Geometry: final body of the model. Coordinates: model frame, mm. Face numbers are marked on the shaded views. A direction names the side the tool comes from. Give positions to 0.01 mm unless a question says otherwise; leave off trailing zeros. Write each loop counter-clockwise with the first axis right and the second up, starting at its lowest first coordinate (ties: lowest second). Pieces come first, ordered by that corner, then holes.
Q1. Mould query, pull axis Z, two halves, no side actions, for the marked faces 6, 7, 8 and 9. Classes: +Z half, -Z half, draft (parallel to the pull), parting line (faces both ways), or undercut.
Q2. Reachability of the marked faces 1, 2, 3, 4 and 5 from +Z, -Z, +X, -X, +Y, -Y: full face, straight path, thin tool, end or side. Return the list, or none.
Q3. Section A-A (x = 26.75). Return the cut outline in (y, z).
Q4. Line query: line 1 (Z direction, x = 23, y = 8.75); line 2 (Z direction, x = 24, y = 20.25); line 3 (Y direction, x = 3.25, z = 5.75). Output: solid intervals per line, ascending.
Q5. Section C-C (x = 17). Return the cut outline in (y, z) (3 decimals).
Q6. Section B-B (y = 2.5). State how many separate pieces and enclosed holes the cut face has, plus the area to 3 significant figures.
Q7. Pin query (flat end, axial travel): pin 1 Ø2 at (y, z) = (16, 3) entering from -X; pin 2 Ø1.5 at (y, z) = (5, 4) entering from +X; pin 3 Ø0.7 at (x, y) = (15.5, 9) entering from -Z. Return the tip coordinate at first contact, or that it passes through.
from build123d import *

# Parameters (mm, degrees)
SKETCH_W             = 28
SKETCH_H             = 22
PAD002_DEPTH         = 5
POCKET001_DEPTH      = 0.8
SKETCH002_W          = 0.6
SKETCH002_H          = 23
POCKET_DEPTH         = 4
LINEARPATTERN_COUNT  = 9
LINEARPATTERN_PITCH  = 2.375
POCKET002_DEPTH      = 3.5
SKETCH006_W          = 28
SKETCH006_H          = 22
POCKET005_DEPTH      = 1
POCKET005_DEPTH_BACK = 1
PAD_DEPTH            = 2


with BuildPart() as part:
    # Sketch → Pad002 (new body)
    with BuildSketch(Plane.XY):
        with Locations((15, 12)):
            Rectangle(SKETCH_W, SKETCH_H)
    extrude(amount=PAD002_DEPTH)

    # Sketch001 → Pocket001 (cut)
    with BuildSketch(Plane.XY):
        with BuildLine():
            ThreePointArc((17.966363, 19.215428), (14.961232, 19.999875), (11.966488, 19.17666))
            Line((11.966488, 19.17666), (4.036475, 13.531422))
            ThreePointArc((4.036475, 13.531422), (3.750333, 12.536475), (4, 11.531754))
            Line((4, 11.531754), (12.33, 5.376817))
            ThreePointArc((12.33, 5.376817), (15.374304, 4.761687), (18.318313, 5.75112))
            Line((18.318313, 5.75112), (26, 11.531754))
            ThreePointArc((26, 11.531754), (26.249667, 12.536475), (25.963525, 13.531422))
            Line((25.963525, 13.531422), (17.966363, 19.215428))
        make_face()
    extrude(amount=POCKET001_DEPTH, mode=Mode.SUBTRACT)

    # Sketch002 → Pocket (cut)
    with BuildSketch(Plane.XY):
        with Locations((6.3, 11.5)):
            Rectangle(SKETCH002_W, SKETCH002_H)
    pocket = extrude(amount=POCKET_DEPTH, mode=Mode.SUBTRACT)

    # LinearPattern: Pocket ×9
    with Locations(*[(i * LINEARPATTERN_PITCH, 0, 0) for i in range(1, LINEARPATTERN_COUNT)]):
        add(pocket, mode=Mode.SUBTRACT)

    # Sketch003 → Pocket002 (cut)
    with BuildSketch(Plane(origin=(0.5, 0, 4), x_dir=(0.707107, 0, -0.707107), z_dir=(0.707107, 0, 0.707107))):
        with BuildLine():
            ThreePointArc((17.966363, 19.215428), (14.961232, 19.999875), (11.966488, 19.17666))
            Line((11.966488, 19.17666), (4.036475, 13.531422))
            ThreePointArc((4.036475, 13.531422), (3.750333, 12.536475), (4, 11.531754))
            Line((4, 11.531754), (12.33, 5.376817))
            ThreePointArc((12.33, 5.376817), (15.374304, 4.761687), (18.318313, 5.75112))
            Line((18.318313, 5.75112), (26, 11.531754))
            ThreePointArc((26, 11.531754), (26.249667, 12.536475), (25.963525, 13.531422))
            Line((25.963525, 13.531422), (17.966363, 19.215428))
        make_face()
    extrude(amount=POCKET002_DEPTH, mode=Mode.SUBTRACT)

    # Sketch006 → Pocket005 (cut, two sides)
    with BuildSketch(Plane.XY.offset(5)) as pocket005_sk:
        with Locations((15, 12)):
            Rectangle(SKETCH006_W, SKETCH006_H)
        with BuildLine():
            ThreePointArc((17.966363, 19.215428), (14.961232, 19.999875), (11.966488, 19.17666))
            Line((11.966488, 19.17666), (4.036475, 13.531422))
            ThreePointArc((4.036475, 13.531422), (3.750333, 12.536475), (4, 11.531754))
            Line((4, 11.531754), (12.33, 5.376817))
            ThreePointArc((12.33, 5.376817), (15.374304, 4.761687), (18.318313, 5.75112))
            Line((18.318313, 5.75112), (26, 11.531754))
            ThreePointArc((26, 11.531754), (26.249667, 12.536475), (25.963525, 13.531422))
            Line((25.963525, 13.531422), (17.966363, 19.215428))
        make_face(mode=Mode.SUBTRACT)
    extrude(amount=-POCKET005_DEPTH, mode=Mode.SUBTRACT)
    extrude(pocket005_sk.sketch, amount=POCKET005_DEPTH_BACK, mode=Mode.SUBTRACT)

    # Sketch004 → Pad (join)
    with BuildSketch(Plane.XY.offset(5)):
        Polygon((5, 19.805), (25, 19.805), (25, 15), (30, 15), (30, 10), (25, 10), (25, 4.805), (5, 4.805), (5, 10), (0, 10), (0, 15), (5, 15), align=None)
    extrude(amount=PAD_DEPTH)


solid = part.part
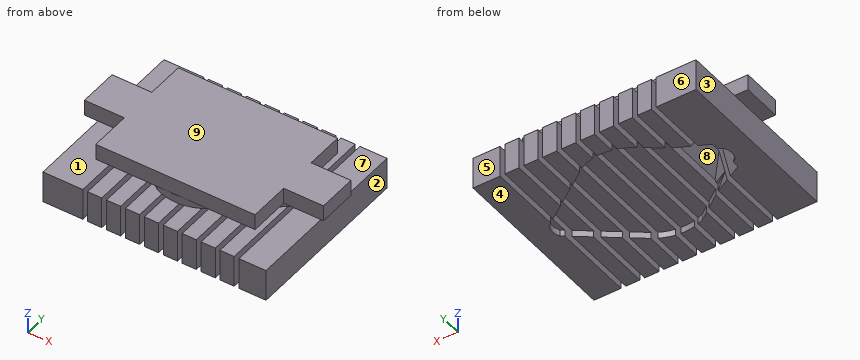
Computed:
1. face 6: draft
1. face 7: undercut
1. face 8: -Z half
1. face 9: +Z half
2. face 1: -X
2. face 2: -Z, +X, +Y, -Y
2. face 3: -Z, -X, +Y, -Y
2. face 4: -Z, +X, -X, +Y, -Y
2. face 5: +Z, -Z, +X, -X, +Y
3. outline: (1, 0) - (23, 0) - (23, 4) - (1, 4) - close; (10, 5) - (15, 5) - (15, 7) - (10, 7) - close
4. line 1: z = 5 to 7
4. line 2: z = 0 to 4
4. line 3: y = 10 to 15
5. outline: (1, 0) - (5.093, 0) - (5.093, 0.8) - (19.657, 0.8) - (19.657, 0) - (23, 0) - (23, 4) - (19.657, 4) - (19.657, 5) - (19.805, 5) - (19.805, 7) - (4.805, 7) - (4.805, 5) - (5.093, 5) - (5.093, 4) - (1, 4) - close
6. separate pieces: 10
6. enclosed holes: 0
6. area: 90.4 mm2
7. pin 1: stops at x = 1
7. pin 2: stops at x = 29
7. pin 3: stops at z = 0.8
